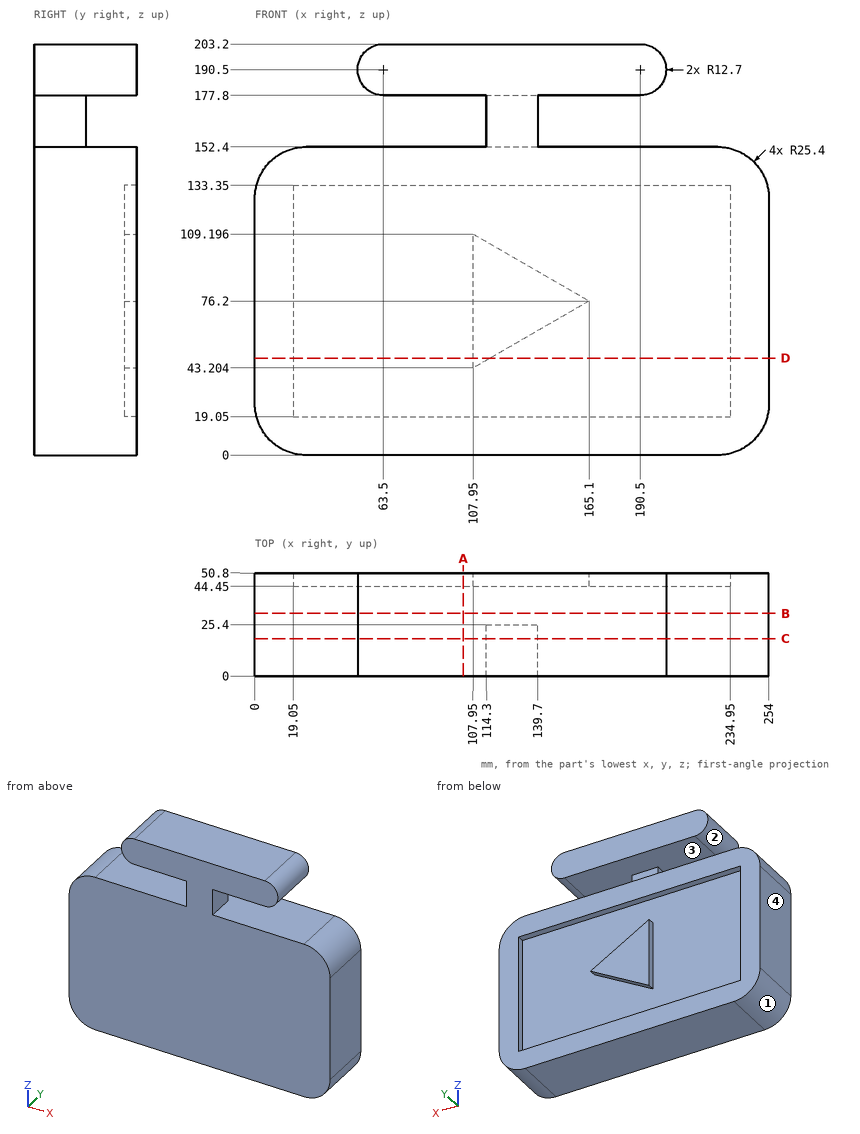
Check sheet for the drawn part. Datum: minimum x, y, z corner. Units: mm. Give positions to 0.01 mm unless a question says otherwise; leave off trailing zeros. Order: outer loops, then holes, each group sorted by start corner. A loop starts at its lowest first (then second) coordinate and runs counter-clockwise, first axis right, second up. Notation, with made-up numbers: (36.5, 6.5) - (89.5, 6.5) arc R12 cw to (89.5, 18.5) - close; hole circle Ø3 at (-12.75, -22). An arc over 180 degrees is marked (long way). Answer as a JSON object with one key per item and string values.
(1) Material ranges on line 1 (Z direction, x = 136, y = 41); line 2 (Y direction, x = 74.5, z = 43); line 3 (Z direction, x = 207, y = 23.5), recorded low to high.
Report:
{"line 1": "0 to 152.4, 177.8 to 203.2", "line 2": "0 to 44.45", "line 3": "0 to 152.4"}
(2) Cross-section at C-C (y = 18.5). Record the cut outline in (x, z), then the cut area to 3 significant figures.
Report:
{"outline": "(0, 25.4) arc R25.4 ccw to (25.4, 0) - (228.6, 0) arc R25.4 ccw to (254, 25.4) - (254, 127) arc R25.4 ccw to (228.6, 152.4) - (139.7, 152.4) - (139.7, 177.8) - (190.5, 177.8) arc R12.7 ccw to (190.5, 203.2) - (63.5, 203.2) arc R12.7 ccw to (63.5, 177.8) - (114.3, 177.8) - (114.3, 152.4) - (25.4, 152.4) arc R25.4 ccw to (0, 127) - close", "area": "42,500 mm^2"}
(3) Draft check along Z on the marked faces 1, 2, 3 and 4. Enter one of: released by +Z, released by -Z, zero draft, split by the parting line, or undercut.
Report:
{"face 1": "released by -Z", "face 2": "undercut", "face 3": "undercut", "face 4": "zero draft"}
(4) Cross-section at D-D (z = 48). Record the cut outline in (x, y).
Report:
{"outline": "(0, 0) - (254, 0) - (254, 50.8) - (234.95, 50.8) - (234.95, 44.45) - (116.26, 44.45) - (116.26, 50.8) - (107.95, 50.8) - (107.95, 44.45) - (19.05, 44.45) - (19.05, 50.8) - (0, 50.8) - close"}
(5) Cross-section at B-B (y = 31). Record the cut outline in (x, z).
Report:
{"outline": "(0, 25.4) arc R25.4 ccw to (25.4, 0) - (228.6, 0) arc R25.4 ccw to (254, 25.4) - (254, 127) arc R25.4 ccw to (228.6, 152.4) - (25.4, 152.4) arc R25.4 ccw to (0, 127) - close; (63.5, 177.8) - (190.5, 177.8) arc R12.7 ccw to (190.5, 203.2) - (63.5, 203.2) arc R12.7 ccw to start"}
(6) Cross-section at A-A (x = 103). Record the cut outline in (y, z).
Report:
{"outline": "(0, 0) - (50.8, 0) - (50.8, 19.05) - (44.45, 19.05) - (44.45, 133.35) - (50.8, 133.35) - (50.8, 152.4) - (0, 152.4) - close; (0, 177.8) - (50.8, 177.8) - (50.8, 203.2) - (0, 203.2) - close"}
(7) Depth check by flat-ended pin: pin 1 Ø12.5 at (y, z) = (16.5, 171) entering from -X; pin 2 Ø12.5 at (y, z) = (18.5, 163) entering from +X; pin 3 Ø12 at (x, z) = (207.5, 164) entering from +Y; pin 4 Ø12.5 at (x, z) = (122.5, 169.5) entering from +Y. Enter the tip coordinate at first touch or a pass-through.
Report:
{"pin 1": "x = 114.3", "pin 2": "x = 139.7", "pin 3": "through", "pin 4": "y = 25.4"}
